Could you check a few things on this model? Use its own coordinates, in mm. Face numbers are marked on the shaded views. A direction names the side the tool comes from. Give positions to 0.01 mm unless a question says otherwise; leave off trailing zeros. Write each loop counter-clockwise with the first axis right and the second up, starting at its lowest first coordinate (ties: lowest second). Pieces come first, ordered by that corner, then holes. Notation, with made-up numbers: M 62.5,38.25 L 106.5,38.25 A25 cw 106.5,69.25 Z; hole C -15.75,19.25 d3. An arc over 180 degrees is marked long. Answer as CSV lines item,"result". Start each with the question number.
from build123d import *

# Parameters (mm, degrees)
SKETCH_1_R          = 13
EXTRUDE_1_DEPTH     = 10
SKETCH_2_W          = 12
SKETCH_2_H          = 60
EXTRUDE_2_DEPTH     = 10
SKETCH_3_R          = 10
CUT_EXTRUDE_1_DEPTH = 10
SKETCH_4_W          = 32.688093459
SKETCH_4_H          = 61.579585558
CUT_EXTRUDE_2_DEPTH = 10


with BuildPart() as part:
    # 草图1 → 凸台-拉伸1 (new body)
    with BuildSketch(Plane(origin=(0, 0, 0), x_dir=(1, 0, 0), z_dir=(0, 1, 0))):
        with Locations(Location((0, 0, 0), (0, 0, 270))):
            Circle(SKETCH_1_R)
    extrude(amount=EXTRUDE_1_DEPTH)

    # 草图2 → 凸台-拉伸2 (add)
    with BuildSketch(Plane(origin=(0, 10, 0), x_dir=(1, 0, 0), z_dir=(0, 1, 0))):
        Rectangle(SKETCH_2_W, SKETCH_2_H)
    extrude(amount=-EXTRUDE_2_DEPTH)

    # 草图3 → 切除-拉伸1 (cut)
    with BuildSketch(Plane(origin=(0, 10, 0), x_dir=(1, 0, 0), z_dir=(0, 1, 0))):
        with Locations(Location((0, 0, 0), (0, 0, 270))):
            Circle(SKETCH_3_R)
    extrude(amount=-CUT_EXTRUDE_1_DEPTH, mode=Mode.SUBTRACT)

    # 草图4 → 切除-拉伸2 (cut)
    with BuildSketch(Plane(origin=(0, 10, 0), x_dir=(1, 0, 0), z_dir=(0, 1, 0))):
        with Locations((13.84404673, -0.789792779)):
            Rectangle(SKETCH_4_W, SKETCH_4_H)
    extrude(amount=-CUT_EXTRUDE_2_DEPTH, mode=Mode.SUBTRACT)


solid = part.part
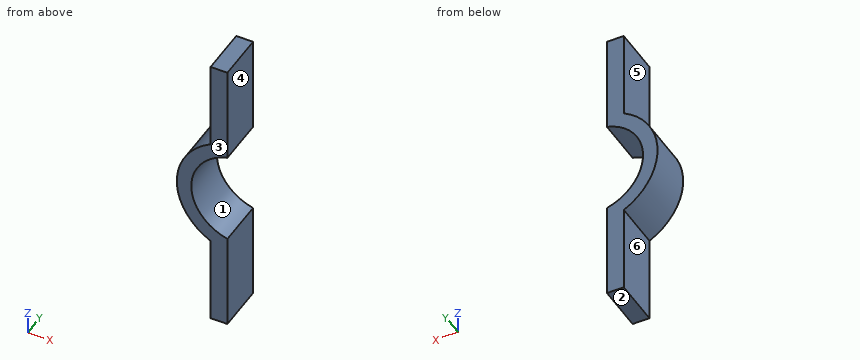
1. Imagine slicing it at B-B, the plane x = -4.5. Please give me the cut outline in (y, z), plus the area to 3 significant figures.
2. Imagine slicing it at D-D, the plane x = -7.75. Please give me the cut outline in (y, z).
3. Please list where these lines run through material, in increasing order: line 1 (X direction, y = 1.5, z = 17); line 2 (Z direction, x = -9, y = 4.5); line 3 (Z direction, x = -8.5, y = 3.5).
4. Imagine slicing it at C-C, the plane z = -26. Please give me the cut outline in (x, y).
5. Imagine slicing it at A-A, the plane y = 3. Please give me the cut outline in (x, z), plus the area to 3 significant figures.
6. Will these pins go through, and if not, where does the flat tip stop? P1, Ø3, axis at y = 7.5, z = 12.5, coming from the -X side; P2, Ø1, axis at y = 2.5, z = -1, coming from the +X side; P3, Ø3, axis at y = 4, z = 18.5, coming from the -X side.
7. On a 3-axis mill with a long thin cutter (end or side, diameter ignored), from which of +Z, -Z, +X, -X, +Y, -Y can I reach the whole of each face in a straight line? I mean the marked faces 4, 5 and 6. Say none if no direction works.
8. Thinking about a two-plate mould opening in Z: for the marked faces 1, 2 and 3, which applies, pulls with the +Z half, pulls with the -Z half, needs draft (parallel to the pull), parting line crosses it, or undercut?
Solutions:
1,outline,"M 0,-30 L 10,-30 L 10,-8.93 L 0,-8.93 Z; M 0,8.93 L 10,8.93 L 10,30 L 0,30 Z"
1,area,"421 mm²"
2,outline,"M 0,-10.44 L 10,-10.44 L 10,-6.32 L 0,-6.32 Z; M 0,6.32 L 10,6.32 L 10,10.44 L 0,10.44 Z"
3,line 1,"-6 to -2.5"
3,line 2,"-9.38 to -4.36, 4.36 to 9.38"
3,line 3,"-9.84 to -5.27, 5.27 to 9.84"
4,outline,"M -6,0 L -2.5,0 L -2.5,10 L -6,10 Z"
5,outline,"M -6,-30 L -2.5,-30 L -2.5,-9.68 A10 cw -2.5,9.68 L -2.5,30 L -6,30 L -6,11.53 A13 ccw -6,-11.53 Z"
5,area,"218 mm²"
6,P1,"x = -6.93"
6,P2,"x = -9.89"
6,P3,"x = -6"
7,face 4,"+Z, -Z, +X, +Y, -Y"
7,face 5,"+Z, -X, +Y, -Y"
7,face 6,"-Z, -X, +Y, -Y"
8,face 1,"undercut"
8,face 2,"pulls with the -Z half"
8,face 3,"needs draft"
